The listing builds one solid part. Answer for the finished solid, in the listing's coordinates (mm). A direction names the side the tool comes from. Give positions to 0.01 mm unless a question says otherwise; leave off trailing zeros. Write each loop counter-clockwise with the first axis right and the second up, starting at its lowest first coordinate (ties: lowest second). Pieces come first, ordered by that corner, then holes. Notation, with made-up numbers: (51.25, 82) - (64.25, 82) arc R30 cw to (64.25, 104) - close; hole circle Ø4 at (-20, 59). An arc over 180 degrees is marked (long way). Return JSON: item names as keys, results as strings.
from build123d import *

# Parameters (mm, degrees)
F0_R     = 1.6
F1_DEPTH = 7.5
F2_R     = 3
F3_W     = 9
F3_H     = 46.435098
F4_DEPTH = 8.001
F6_D     = 3.2


with BuildPart() as f1:
    # F0 (on Right) → F1 (new body, symmetric)
    with BuildSketch(Plane.YZ):
        with BuildLine():
            ThreePointArc((3, 0), (0, 3), (-3, 0))
            Line((-3, 0), (-3, -5))
            Line((-3, -5), (-7.5, -5))
            Line((-7.5, -5), (-7.5, -7.5))
            Line((-7.5, -7.5), (7.5, -7.5))
            Line((7.5, -7.5), (7.5, -5))
            Line((7.5, -5), (3, -5))
            Line((3, -5), (3, 0))
        make_face()
        Circle(F0_R, mode=Mode.SUBTRACT)
    extrude(amount=F1_DEPTH, both=True)

    # F2
    f2_edges = [f1.edges().sort_by_distance(p)[0] for p in [
        (0, -3, -5),
        (0, 3, -5),
    ]]
    fillet(f2_edges, radius=F2_R)

    # F3 (on face) → F4 (cut, through all)
    with BuildSketch(Plane.XY.offset(-5)):
        Rectangle(F3_W, F3_H)
    extrude(amount=F4_DEPTH, mode=Mode.SUBTRACT)

    # F6 (through all)
    with Locations(Plane.XY):
        with Locations((0, 0)):
            Hole(F6_D / 2)


solid = f1.part
Item 1: Consider L1, parallel to Z at x = -6.2, y = 0; L2, parallel to Y at x = 5.45, z = 0; L3, parallel to X at y = 0.5, z = 1.75. Determine where each line is inside the solid, lowest interval first.
Answer below:
{"L1": "z = -7.5 to -1.6, 1.6 to 3", "L2": "y = -3 to -1.6, 1.6 to 3", "L3": "x = -7.5 to -4.5, 4.5 to 7.5"}
Item 2: A cutting plane is placed at D-D on z = -0.75. Determine the outline of the cut face in (x, y), then the cut area to 3 significant figures.
Answer below:
{"outline": "(-7.5, -3) - (-4.5, -3) - (-4.5, -1.41) - (-7.5, -1.41) - close; (-7.5, 1.41) - (-4.5, 1.41) - (-4.5, 3) - (-7.5, 3) - close; (4.5, -3) - (7.5, -3) - (7.5, -1.41) - (4.5, -1.41) - close; (4.5, 1.41) - (7.5, 1.41) - (7.5, 3) - (4.5, 3) - close", "area": "19.0 mm²"}
Item 3: For faces 1 (the face through (7.5, 0, -5)), 2 (the face through (6, 3, -1)), 3 (the face through (-6, -3, -1)), determine the directions among +Z, -Z, +X, -X, +Y, -Y from which every point of the face is accessible in a straight line to the end or side of a thin tool.
Answer below:
{"face 1": "+Z, -Z, +X, +Y, -Y", "face 2": "+Z, +X, -X, +Y", "face 3": "+Z, +X, -X, -Y"}
Item 4: The mould has two halves that part along Z. Classify faces 4 (the face through (0, -2, -7.5)), 5 (the face through (-6, 0, 3)), 6 (the face through (-6.02, -1.27, -0.97)), 7 (the face through (-6, 3, -1)): +Z half, -Z half, draft (parallel to the pull), parting line (faces both ways), or undercut.
Answer below:
{"face 4": "-Z half", "face 5": "+Z half", "face 6": "undercut", "face 7": "draft"}
Item 5: A cutting plane is placed at B-B on y = 0. Determine the outline of the cut face in (x, z).
Answer below:
{"outline": "(-7.5, -7.5) - (-1.6, -7.5) - (-1.6, -5) - (-4.5, -5) - (-4.5, -1.6) - (-7.5, -1.6) - close; (-7.5, 1.6) - (-4.5, 1.6) - (-4.5, 3) - (-7.5, 3) - close; (1.6, -7.5) - (7.5, -7.5) - (7.5, -1.6) - (4.5, -1.6) - (4.5, -5) - (1.6, -5) - close; (4.5, 1.6) - (7.5, 1.6) - (7.5, 3) - (4.5, 3) - close"}
Item 6: Flat-ended cylindrical pins translate along their axes: P1, Ø5, axis at y = 5, z = 1.5, coming from the +X side; P2, Ø2.5, axis at x = 0, y = 0, coming from the +Z side; P3, Ø1.6, axis at x = -6, z = -1.5, coming from the -Y side; P4, Ø5, axis at x = 3, z = 0.5, coming from the +Y side. Find the tip coordinate at first contact, or state that the pin passes through.
Answer below:
{"P1": "stops at x = 7.5", "P2": "passes through", "P3": "stops at y = -3.02", "P4": "stops at y = 3"}
Item 7: A cutting plane is placed at A-A on x = 0. Determine the outline of the cut face in (y, z).
Answer below:
{"outline": "(-7.5, -7.5) - (-1.6, -7.5) - (-1.6, -5) - (-7.5, -5) - close; (1.6, -7.5) - (7.5, -7.5) - (7.5, -5) - (1.6, -5) - close"}
Item 8: A cutting plane is placed at C-C on z = -2.25. Determine the outline of the cut face in (x, y).
Answer below:
{"outline": "(-7.5, -3.01) - (-4.5, -3.01) - (-4.5, 3.01) - (-7.5, 3.01) - close; (4.5, -3.01) - (7.5, -3.01) - (7.5, 3.01) - (4.5, 3.01) - close"}
